Could you check a few things on this model? Use its own coordinates, in mm. A direction names the side the tool comes from. Coordinates: 2 decimals unless noted, no trailing zeros. Order: outer loops, then holes, each group sorted by start corner. A loop starts at its lowest first (then second) coordinate and runs counter-clockwise, first axis right, second up. Notation, with made-up numbers: (81.5, 21) - (118.5, 21) arc R15 ccw to (118.5, 27) - close; hole circle Ø6 at (72.25, -21). An arc over 180 degrees is marked (long way). Answer as a JSON object with one key per item and string values. Group by question number.
(1) We'd pull the mould along Y, two halves only. Please class faces 1 (the cylindrical face through (64.37, -60.97, 9.3)), 2 (the cylindrical face through (74.651, -4.868, 9.297)), 3 (the flat face through (-81, 0, 25)): pulls with the +Y half, pulls with the -Y half, needs draft (parallel to the pull), parting line crosses it, or undercut.
(2) Will these pins go through, and if not, where does the flat tip stop? P1, Ø2, axis at y = 85.5, z = 7, coming from the +X side; P2, Ø8, axis at y = -72, z = 9, coming from the +X side (3 decimals); P3, Ø5, axis at x = -82.5, y = -45.5, coming from the -Z side.
(3) Please list where these lines run through material, in increasing order: probe 1 along Z at (x, y) = (75, -66); probe 2 along Z at (x, y) = (-18, -19); probe 3 along X at (y, z) = (3, -6.5).
(4) Imagine slicing it at D-D, the plane y = -38.5. Write out the boundary of the cut face in (x, z).
(5) Imagine slicing it at A-A, the plane y = 0. Write out the boundary of the cut face in (x, z), and give its area (3 significant figures).
(6) Imagine slicing it at C-C, the plane z = -38.5. Write out the boundary of the cut face in (x, y).
(7) Which directions (+Z, -Z, +X, -X, +Y, -Y) give clear straight access to the entire face, cutting with the end or side of a thin tool? Please do faces 4 (the flat face through (0, -81, 25)), 5 (the cylindrical face through (-29.97, -1.32, -52.18)), 6 (the cylindrical face through (0, 73, 9)).
from build123d import *

# Parameters (mm, degrees)
SKETCH2_R                    = 8
BOSS_EXTRUDE1_DEPTH          = 30
CHAMFER1_SIZE                = 1
CIRPATTERN1_COUNT            = 8
CHAMFER1_OF_CIRPATTERN1_SIZE = 1


with BuildPart() as part:
    # Sketch1 → Revolve1 (revolve)
    with BuildSketch(Plane(origin=(0, 0, 0), x_dir=(1, 0, 0), z_dir=(0, 1, 0))):
        Polygon((0, 0), (0, 75), (30, 75), (30, 30), (109, 30), (109, 5), (53, 5), (53, 0), align=None)
    revolve(axis=Axis((0, 0, 0), (0, 0, -1)))

    # Sketch2 → Boss-Extrude1 (add)
    with BuildSketch(Plane.XY.offset(-5)):
        with Locations((81, 0)):
            Circle(SKETCH2_R)
    boss_extrude1 = extrude(amount=BOSS_EXTRUDE1_DEPTH)

    # Chamfer1
    chamfer1_edges = [part.edges().sort_by_distance(p)[0] for p in [
        (73, 0, 25),
    ]]
    chamfer(chamfer1_edges, length=CHAMFER1_SIZE)

    # CirPattern1: Boss-Extrude1 ×8 about axis
    cirpattern1_axis = Axis((0, 0, 0), (0, 0, 1))
    for i in range(1, CIRPATTERN1_COUNT):
        add(boss_extrude1.rotate(cirpattern1_axis, i * 360 / CIRPATTERN1_COUNT))

    # Chamfer1 of CirPattern1
    chamfer1_of_cirpattern1_edges = [part.edges().sort_by_distance(p)[0] for p in [
        (51.618795027, 51.618795027, 25),
        (0, 73, 25),
        (-51.618795027, 51.618795027, 25),
        (-73, 0, 25),
        (-51.618795027, -51.618795027, 25),
        (0, -73, 25),
        (51.618795027, -51.618795027, 25),
    ]]
    chamfer(chamfer1_of_cirpattern1_edges, length=CHAMFER1_OF_CIRPATTERN1_SIZE)


solid = part.part
Result set:
{
 "1": {"face 1": "undercut", "face 2": "parting line crosses it", "face 3": "needs draft"},
 "2": {"P1": "stops at x = 7.19", "P2": "stops at x = 6.245", "P3": "stops at z = -30"},
 "3": {"probe 1": "z = -30 to -5", "probe 2": "z = -75 to 0", "probe 3": "x = -108.96 to 108.96"},
 "4": {"outline": "(-101.97, -30) - (101.97, -30) - (101.97, -5) - (36.42, -5) - (36.42, 0) - (-36.42, 0) - (-36.42, -5) - (-101.97, -5) - close"},
 "5": {"outline": "(-109, -30) - (-30, -30) - (-30, -75) - (30, -75) - (30, -30) - (109, -30) - (109, -5) - (89, -5) - (89, 24) - (88, 25) - (74, 25) - (73, 24) - (73, -5) - (53, -5) - (53, 0) - (-53, 0) - (-53, -5) - (-73, -5) - (-73, 24) - (-74, 25) - (-88, 25) - (-89, 24) - (-89, -5) - (-109, -5) - close", "area": "9,640 mm^2"},
 "6": {"outline": "circle Ø60 at (0, 0)"},
 "7": {"face 4": "+Z, +X, -X, +Y, -Y", "face 5": "-Z", "face 6": "+Z"}
}
